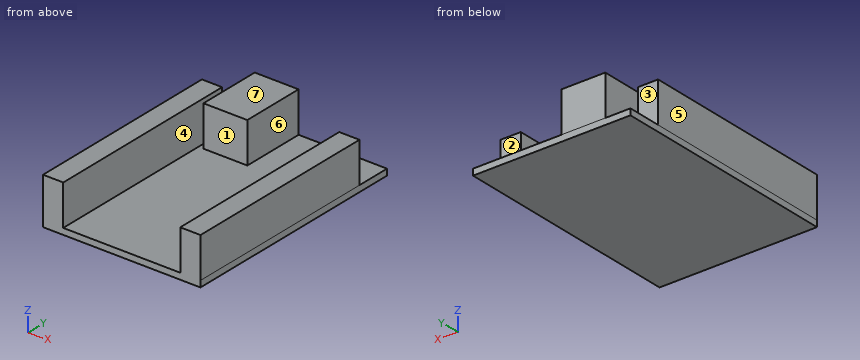
from build123d import *

# Parameters (mm, degrees)
F0_W     = 40.5
F0_H     = 60
F1_DEPTH = 1.6
F2_W     = 5.203603
F2_H     = 51.121294
F2_W_2   = 11.289145
F2_H_2   = 16.489763
F3_DEPTH = 12


with BuildPart() as f1:
    # F0 (on Top) → F1 (new body)
    with BuildSketch(Plane.XY):
        with Locations((20.25, 30)):
            Rectangle(F0_W, F0_H)
    extrude(amount=F1_DEPTH)

    # F2 (on Top) → F3 (join)
    with BuildSketch(Plane.XY):
        with Locations((2.601802, 25.560647)):
            Rectangle(F2_W, F2_H)
        with Locations((37.898198, 25.560647)):
            Rectangle(F2_W, F2_H)
        with Locations((12.116618, 51.755118)):
            Rectangle(F2_W_2, F2_H_2)
    extrude(amount=F3_DEPTH)


solid = f1.part
Source: CAD feature listing. Evaluate the final solid. Frame: model axes, mm. Face numbers are marked on the shaded views. A direction names the side the tool comes from. Coordinates: 2 decimals unless noted, no trailing zeros. Loops run counter-clockwise (first coordinate to the right, second up) from the corner with the lowest first, then second, coordinate; pieces in that order, holes last. Notation, with made-up numbers: (21, -29) - (46, -29) arc R25 cw to (46, -15) - close; hole circle Ø10 at (36.25, 69.25). An arc over 180 degrees is marked (long way). Return JSON: item names as keys, results as strings.
Q1. Section A-A, the plane z = 6.25. Return loops of the section in (x, y).
Results:
{"outline": "(0, 0) - (5.2, 0) - (5.2, 51.12) - (0, 51.12) - close; (6.47, 43.51) - (17.76, 43.51) - (17.76, 60) - (6.47, 60) - close; (35.3, 0) - (40.5, 0) - (40.5, 51.12) - (35.3, 51.12) - close"}
Q2. Section B-B, the plane y = 40.5. Return loops of the section in (x, z).
Results:
{"outline": "(0, 0) - (40.5, 0) - (40.5, 12) - (35.3, 12) - (35.3, 1.6) - (5.2, 1.6) - (5.2, 12) - (0, 12) - close"}
Q3. Mould query, pull axis X, two halves, no side actions, for the marked faces 5, 6 and 7. Classes: released by +X, released by -X, zero draft, split by the parting line, or undercut.
Results:
{"face 5": "released by -X", "face 6": "undercut", "face 7": "zero draft"}
Q4. Access query for the marked faces 1, 2, 3 and 4. Directions: +Z, -Z, +X, -X, +Y, -Y. A direction counts if a zero-diameter tool reaches every point of the face in a straight line with its end or side. Return the directions, or none.
Results:
{"face 1": "+Z, -Y", "face 2": "+Z, +X, +Y", "face 3": "+Z, -X, +Y", "face 4": "+Z, +Y, -Y"}
Q5. Section C-C, the plane x = 10. Return loops of the section in (y, z).
Results:
{"outline": "(0, 0) - (60, 0) - (60, 12) - (43.51, 12) - (43.51, 1.6) - (0, 1.6) - close"}
Q6. Contact query for flat-ended pins moving along their axis: P1, Ø12, axis at x = 20.5, y = 21.5, coming from the -Z side; P2, Ø5, axis at x = 11.5, z = 9, coming from the -Y side; P3, Ø3, axis at x = 21, z = 5, coming from the +Y side; P4, Ø2.5, axis at x = 1.5, z = 8, coming from the +Y side. Output: stop coordinate, or through.
Results:
{"P1": "z = 0", "P2": "y = 43.51", "P3": "through", "P4": "y = 51.12"}
Q7. Section D-D, the plane y = 52. Return loops of the section in (x, z), plus the area to 3 significant figures.
Results:
{"outline": "(0, 0) - (40.5, 0) - (40.5, 1.6) - (17.76, 1.6) - (17.76, 12) - (6.47, 12) - (6.47, 1.6) - (0, 1.6) - close", "area": "182 mm2"}
Q8. Material intervals for line 1 along X through (y, z) = (49, 8); line 2 along X through (y, z) = (10, 3.75); line 3 along Z through (x, y) = (33, 43), sorted ascending.
Results:
{"line 1": "0 to 5.2, 6.47 to 17.76, 35.3 to 40.5", "line 2": "0 to 5.2, 35.3 to 40.5", "line 3": "0 to 1.6"}
